Job drawing, mm, ordinate dimensions from the low corner. One solid piece. Coordinates: 2 decimals unless noted, no trailing zeros. Loops run counter-clockwise (first coordinate to the right, second up) from the corner with the lowest first, then second, coordinate; pieces in that order, holes last. Notation, with made-up numbers: M -1.5,77 L 56.5,77 A3 ccw 56.5,81 Z; hole C -28,-27.75 d11. An arc over 180 degrees is marked long. Answer as a JSON object with one key per item and string values. Group by question number.
1. Drill centre lines: L1, parallel to Z at x = 24.5, y = 7.75; L2, parallel to Y at x = 329.5, z = 10.5 (1 decimal). Where is each one in solid material? Low to high.
2. Saw through at A-A on y = 7.75. Write the cut outline in (x, z), then the cut area to 3 significant figures.
3. Drop flat-ended pins along their axis: pin 1 Ø1 at (y, z) = (5, 4.5) entering from -X; pin 2 Ø1 at (x, z) = (150.5, 9) entering from +Y (1 decimal). Give the stop position or say it passes through.
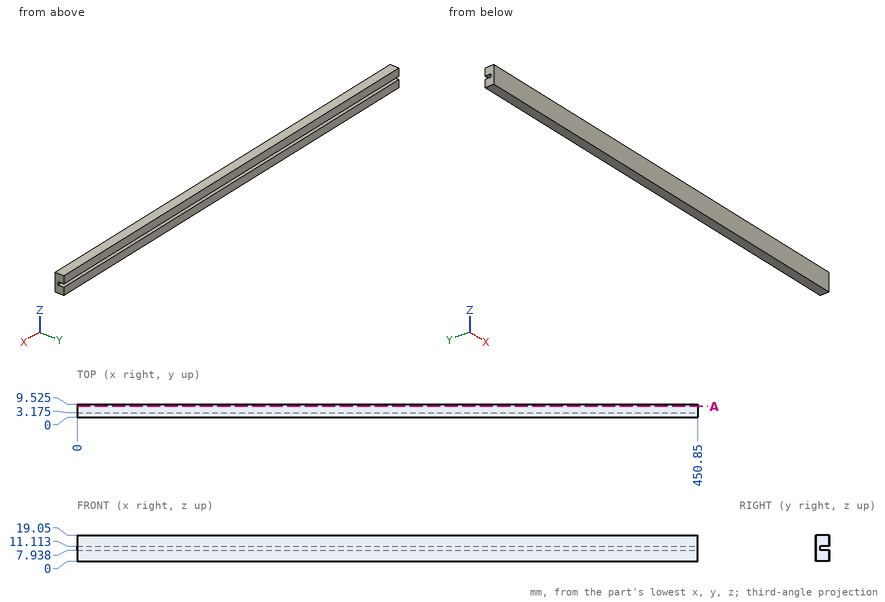
Outcome:
{
 "1": {"L1": "z = 0 to 7.94, 11.11 to 19.05", "L2": "y = 0 to 3.2"},
 "2": {"outline": "M 0,0 L 450.85,0 L 450.85,7.94 L 0,7.94 Z; M 0,11.11 L 450.85,11.11 L 450.85,19.05 L 0,19.05 Z", "area": "7,160 mm²"},
 "3": {"pin 1": "stops at x = 0", "pin 2": "stops at y = 3.2"}
}
